Could you check a few things on this model? Use its own coordinates, in mm. Face numbers are marked on the shaded views. A direction names the side the tool comes from. Give positions to 0.01 mm unless a question says otherwise; leave off trailing zeros. Loops run counter-clockwise (first coordinate to the right, second up) from the corner with the lowest first, then second, coordinate; pieces in that order, holes last. Notation, with made-up numbers: M 6.5,-34 L 38.5,-34 A14 ccw 38.5,-14 Z; hole C 87,1.25 d9. An arc over 180 degrees is marked long. Return JSON: item names as keys, results as strings. Group by question number.
1. Please list where these lines run through material, in increasing order: line 1 (X direction, y = -11.5, z = -1.25); line 2 (X direction, y = -10.25, z = -0.6); line 3 (Y direction, x = -14, z = -0.05).
2. If we section it at D-D (x = 22): Write out the boundary of the cut face in (y, z), plus the area to 3 significant figures.
3. For the marked faces 3 and 4, which set-ups out of +Z, -Z, +X, -X, +Y, -Y let a thin tool reach every point of the face, with its end or its side?
4. For pin 1 (11 mm diameter, centred on x = -12.32, y = -7.51, fed in from +Z), with a flat end and sliding along its axis, tell me the tip position at first contact or that it passes through.
5. If we section it at C-C (y = 8.75): Write out the boundary of the cut face in (x, z).
6. If we section it at B-B (x = -14): Write out the boundary of the cut face in (y, z).
7. If we section it at A-A (z = -0.8): Write out the boundary of the cut face in (x, y).
8. If we mould it in two halves opening along Y, with no side actions, what happens to the marked faces 1 and 2? For each: +Y half, -Y half, draft (parallel to the pull), parting line (faces both ways), or undercut.
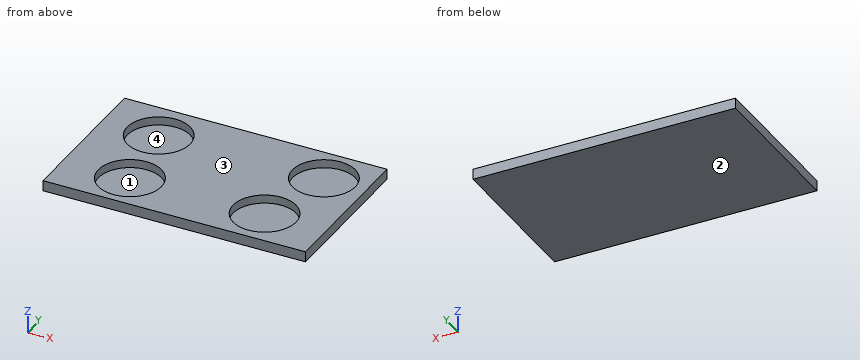
```python
from build123d import *

# Parameters (mm, degrees)
F0_W     = 50
F0_H     = 30
F1_DEPTH = 2
F2_R     = 6
F3_DEPTH = 1.6


with BuildPart() as f1:
    # F0 (on Top) → F1 (new body)
    with BuildSketch(Plane.XY):
        Rectangle(F0_W, F0_H)
    extrude(amount=-F1_DEPTH)

    # F2 (on Top) → F3 (cut)
    with BuildSketch(Plane.XY):
        with Locations((-14.305306, 6.940198)):
            Circle(F2_R)
        with Locations((-12.322392, -7.506745)):
            Circle(F2_R)
        with Locations((13.172213, -7.223471)):
            Circle(F2_R)
        with Locations((16.854765, 7.506745)):
            Circle(F2_R)
    extrude(amount=-F3_DEPTH, mode=Mode.SUBTRACT)


solid = f1.part
```
Answer:
{
 "1": {"line 1": "x = -25 to -16.8, -7.84 to 8.96, 17.38 to 25", "line 2": "x = -25 to -17.66, -6.99 to 7.99, 18.35 to 25", "line 3": "y = -15 to -13.27, -1.75 to 0.95, 12.93 to 15"},
 "2": {"outline": "M -15,-2 L 15,-2 L 15,0 L 10.59,0 L 10.59,-1.6 L 4.42,-1.6 L 4.42,0 L -15,0 Z", "area": "50.1 mm²"},
 "3": {"face 3": "+Z, +X, -X, +Y, -Y", "face 4": "+Z"},
 "4": {"pin 1": "stops at z = -1.6"},
 "5": {"outline": "M -25,-2 L 25,-2 L 25,0 L 22.72,0 L 22.72,-1.6 L 10.98,-1.6 L 10.98,0 L -8.58,0 L -8.58,-1.6 L -20.03,-1.6 L -20.03,0 L -25,0 Z"},
 "6": {"outline": "M -15,-2 L 15,-2 L 15,0 L 12.93,0 L 12.93,-1.6 L 0.95,-1.6 L 0.95,0 L -1.75,0 L -1.75,-1.6 L -13.27,-1.6 L -13.27,0 L -15,0 Z"},
 "7": {"outline": "M -25,-15 L 25,-15 L 25,15 L -25,15 Z; hole C -14.31,6.94 d12; hole C -12.32,-7.51 d12; hole C 13.17,-7.22 d12; hole C 16.85,7.51 d12"},
 "8": {"face 1": "undercut", "face 2": "draft"}
}
